The drawing under review shows one solid part. Ordinate dimensions are in mm from its lowest x, y, z. A direction names the side the tool comes from. Coordinates: 2 decimals unless noted, no trailing zeros. Write each loop counter-clockwise with the first axis right and the second up, starting at its lowest first coordinate (ties: lowest second). Pieces come first, ordered by that corner, then holes. Notation, with made-up numbers: M -20,-9.75 L 33,-9.75 A20 ccw 33,7.25 Z; hole C 78.5,-27 d4. An arc over 180 degrees is marked long. Answer as CSV lines item,"result". Start each with the question number.
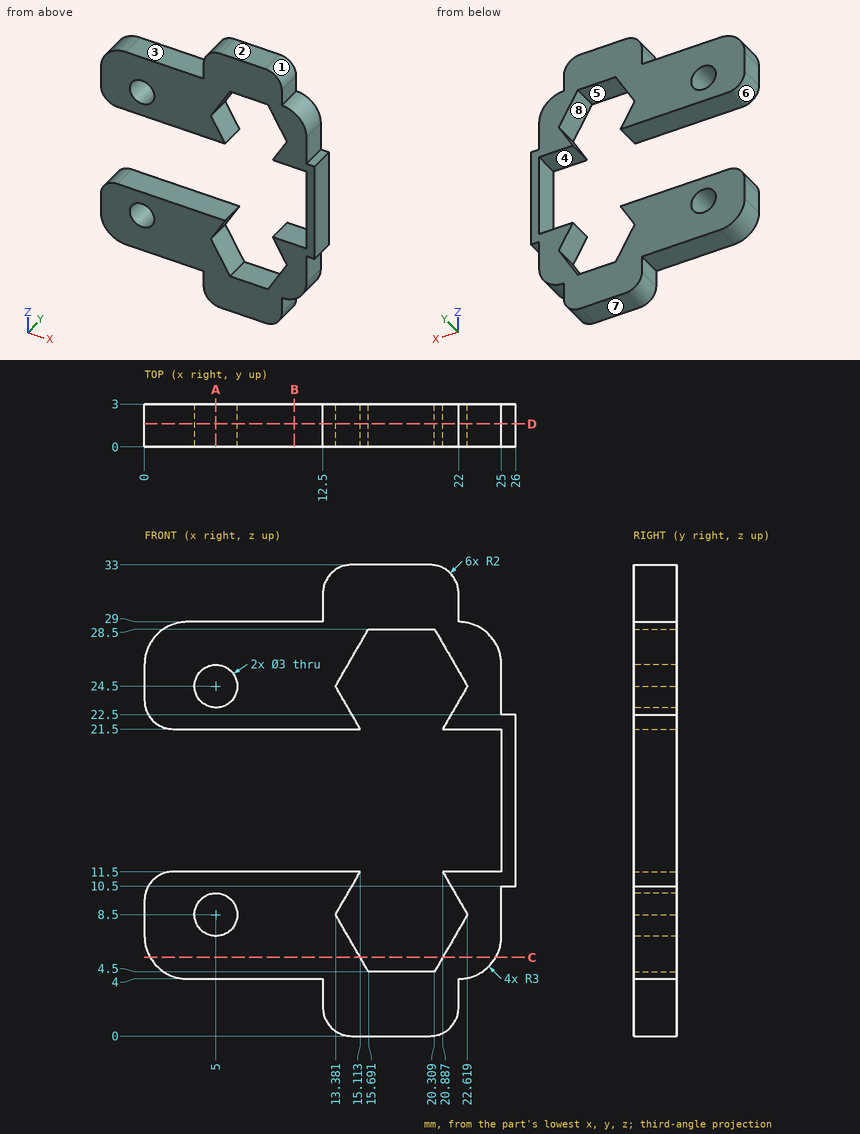
1) Tool access review of the marked faces 1, 2, 3, 4 and 5: name each direction out of +Z, -Z, +X, -X, +Y, -Y from which nothing blocks a thin tool from reaching the whole face with its end or side.
2) Mouldability with a two-part tool opening along X and no side actions: class the marked faces 6, 7 and 8 as +X half, -X half, draft (parallel to the pull), parting line (faces both ways), or undercut.
3) Clearance check with flat-ended pins moving along their axes: pin 1 Ø0.6 at (y, z) = (2, 3) entering from +X; pin 2 Ø0.9 at (x, y) = (23.5, 1) entering from -Z; pin 3 Ø1.6 at (y, z) = (2, 3) entering from -X; pin 4 Ø1.5 at (x, z) = (23, 18.5) entering from +Y. State where each tip first meets the part, or that it passes through.
4) Take a section at D-D on y = 1.6. Give the number of separate pieces and of enclosed holes in the cut face.
5) To check wall thickness, follow line 1 (Z direction, x = 5, y = 2.35); line 2 (Z direction, x = 7.5, y = 1.65); line 3 (Z direction, x = 16, y = 1). State the ranges of each line that lie inside material, in increasing order. Write a range as [from, to].
6) Take a section at C-C on z = 5.5. Give the boundary of the cut face in (x, y).
7) Take a section at A-A on x = 5. Give the boundary of the cut face in (y, z).
8) Take a section at B-B on x = 10.5. Give the boundary of the cut face in (y, z), and give its area (3 significant figures).
Results:
1,face 1,"+Z, +X, +Y, -Y"
1,face 2,"+Z, +X, -X, +Y, -Y"
1,face 3,"+Z, -X, +Y, -Y"
1,face 4,"-X, +Y, -Y"
1,face 5,"+Y, -Y"
2,face 6,"-X half"
2,face 7,"draft"
2,face 8,"undercut"
3,pin 1,"stops at x = 22"
3,pin 2,"stops at z = 4.19"
3,pin 3,"stops at x = 12.5"
3,pin 4,"passes through"
4,separate pieces,"1"
4,enclosed holes,"2"
5,line 1,"z = [4, 7], [10, 11.5], [21.5, 23], [26, 29]"
5,line 2,"z = [4, 11.5], [21.5, 29]"
5,line 3,"z = [0, 4.5], [28.5, 33]"
6,outline,"M 0.4,0 L 15.11,0 L 15.11,3 L 0.4,3 Z; M 20.89,0 L 24.6,0 L 24.6,3 L 20.89,3 Z"
7,outline,"M 0,4 L 3,4 L 3,7 L 0,7 Z; M 0,10 L 3,10 L 3,11.5 L 0,11.5 Z; M 0,21.5 L 3,21.5 L 3,23 L 0,23 Z; M 0,26 L 3,26 L 3,29 L 0,29 Z"
8,outline,"M 0,4 L 3,4 L 3,11.5 L 0,11.5 Z; M 0,21.5 L 3,21.5 L 3,29 L 0,29 Z"
8,area,"45.0 mm²"
